from build123d import *

# Parameters (mm, degrees)
BOSS_EXTRUDE1_DEPTH   = 89.408
SKETCH2_W             = 64.008
SKETCH2_H             = 76.2
CUT_EXTRUDE1_DEPTH    = 178.146381459
F_7_0MM_DOWEL_HOLE1_D = 7
FILLET1_R             = 6.35


with BuildPart() as part:
    # Sketch1 → Boss-Extrude1 (new body)
    with BuildSketch(Plane(origin=(0, 0, 0), x_dir=(0, 0, -1), z_dir=(1, 0, 0))):
        Polygon((0, 0), (-114.3, 0), (-114.3, 50.8), (-25.4, 50.8), (-25.4, 101.6), (0, 101.6), align=None)
    extrude(amount=BOSS_EXTRUDE1_DEPTH)

    # Sketch2 → Cut-Extrude1 (cut, through all)
    with BuildSketch(Plane(origin=(0, 0, 0), x_dir=(-1, 0, 0), z_dir=(0, 0, -1))):
        with Locations((-44.704, 38.1)):
            Rectangle(SKETCH2_W, SKETCH2_H)
    extrude(amount=-CUT_EXTRUDE1_DEPTH, mode=Mode.SUBTRACT)

    # Ø7.0mm Dowel Hole1 (through all)
    with Locations(Plane(origin=(0, 101.6, 0), x_dir=(1, 0, 0), z_dir=(0, 1, 0))):
        with Locations((44.704, -12.7)):
            Hole(F_7_0MM_DOWEL_HOLE1_D / 2)

    # Fillet1
    fillet1_edges = [part.edges().sort_by_distance(p)[0] for p in [
        (83.058, 50.8, 25.4),
        (6.35, 50.8, 25.4),
        (76.708, 76.2, 12.7),
        (12.7, 76.2, 12.7),
        (0, 101.6, 12.7),
        (89.408, 101.6, 12.7),
    ]]
    fillet(fillet1_edges, radius=FILLET1_R)


solid = part.part
Input: part model. Units: mm. Frame: model coordinates. A direction names the side the tool comes from. Coordinates: 2 decimals unless noted, no trailing zeros. Loops run counter-clockwise (first coordinate to the right, second up) from the corner with the lowest first, then second, coordinate; pieces in that order, holes last. Notation, with made-up numbers: (83, 30) -> (115, 30) arc R19 cw to (115, 57) -> close; hole circle Ø1 at (35.25, 59.25). An arc over 180 degrees is marked (long way). Write each question's results on one line, items separated by ' | '. Start each with the question number.
Q1. Pin query (flat end, axial travel): pin 1 (8 mm diameter, centred on x = 77, z = 46, fed in from +Y); pin 2 (9 mm diameter, centred on x = 44.704, z = 12.7, fed in from -Y). Return the tip coordinate at first contact, or that it passes through.
Q2. Section D-D, the plane x = 29. Return the cut outline in (y, z), plus the area to 3 significant figures.
Q3. Section A-A, the plane z = 77. Return the cut outline in (x, y).
Q4. Section C-C, the plane z = 7. Return the cut outline in (x, y).
Q5. Section B-B, the plane y = 20.5. Return the cut outline in (x, z).
Q6. Ray query, line 1 (X direction, y = 81.75, z = 12.7); line 2 (X direction, y = 48, z = 18.5); line 3 (Y direction, x = 81.5, z = 54.5). Return the intervals inside material, ascending. Write a range as from..to.
Q7. Reachability of faces 4 (the flat face through (83, 25, 114.3)), 5 (the flat face through (12.7, 27, 56)), 6 (the flat face through (44, 84, 25.4)) from +Z, -Z, +X, -X, +Y, -Y: full face, straight path, thin tool, end or side. Return the list, or none.
Q8. Pull-direction query (Z, two-part tool) for faces 1 (the flat face through (76.708, 27, 56)), 2 (the cylindrical face through (41.366, 88.722, 11.649)), 3 (the flat face through (6, 25, 114.3)); classes: released by +Z, released by -Z, zero draft, split by the parting line, or undercut.
Found:
1) pin 1: y = 50.8 | pin 2: y = 76.2
2) outline: (76.2, 0) -> (101.6, 0) -> (101.6, 25.4) -> (76.2, 25.4) -> close | area: 645 mm2
3) outline: (0, 0) -> (12.7, 0) -> (12.7, 50.8) -> (0, 50.8) -> close; (76.71, 0) -> (89.41, 0) -> (89.41, 50.8) -> (76.71, 50.8) -> close
4) outline: (0, 0) -> (12.7, 0) -> (12.7, 69.85) arc R6.35 cw to (19.05, 76.2) -> (70.36, 76.2) arc R6.35 cw to (76.71, 69.85) -> (76.71, 0) -> (89.41, 0) -> (89.41, 95.25) arc R6.35 ccw to (83.06, 101.6) -> (6.35, 101.6) arc R6.35 ccw to (0, 95.25) -> close
5) outline: (0, 0) -> (12.7, 0) -> (12.7, 114.3) -> (0, 114.3) -> close; (76.71, 0) -> (89.41, 0) -> (89.41, 114.3) -> (76.71, 114.3) -> close
6) line 1: 0..41.2, 48.2..89.41 | line 2: 0..12.7, 76.71..89.41 | line 3: 0..50.8
7) face 4: +Z, +X, -X, +Y, -Y | face 5: +Z, -Z, -Y | face 6: +Z, +X, -X, +Y
8) face 1: zero draft | face 2: undercut | face 3: released by +Z
